Geometry: see drawing. Coordinates: mm, zero at the bounding-box minimum. A direction names the side the tool comes from. Coordinates: 2 decimals unless noted, no trailing zeros. Loops run counter-clockwise (first coordinate to the right, second up) from the corner with the lowest first, then second, coordinate; pieces in that order, holes last. Notation, with made-up numbers: (56.5, 32) -> (67.5, 32) arc R33 ccw to (67.5, 65) -> close; hole circle Ø10 at (-29, -24). An arc over 180 degrees is marked (long way). Put each result on its own line as item: value. Start each with the question number.
1) Contact query for flat-ended pins moving along their axis: P1, Ø1, axis at x = 2.5, z = 4, coming from the +Y side; P2, Ø1, axis at y = 3.5, z = 27, coming from the +X side; P3, Ø2, axis at x = 1, z = 13.5, coming from the -Y side; P4, Ø1, axis at y = 3, z = 24.5, coming from the -X side. Output: stop coordinate, or through.
2) Cut plane B-B (z = 9). Return the cut outline in (x, y).
3) Cut plane C-C (y = 3.85). Return the cut outline in (x, z).
4) Set-up query: the marked faces 1, 2 and 3. Return all of +Z, -Z, +X, -X, +Y, -Y with unobstructed straight access to the full face (end or side cutting, diameter ignored); none if empty.
5) Cut plane A-A (x = 2.65). Return the cut outline in (y, z).
6) Material intervals for L1, parallel to Z at x = 2.7, y = 5.1; L2, parallel to X at y = 4.5, z = 30, sorted ascending.
7) Cut plane D-D (x = 4.05). Return the cut outline in (y, z), plus the area to 3 significant figures.
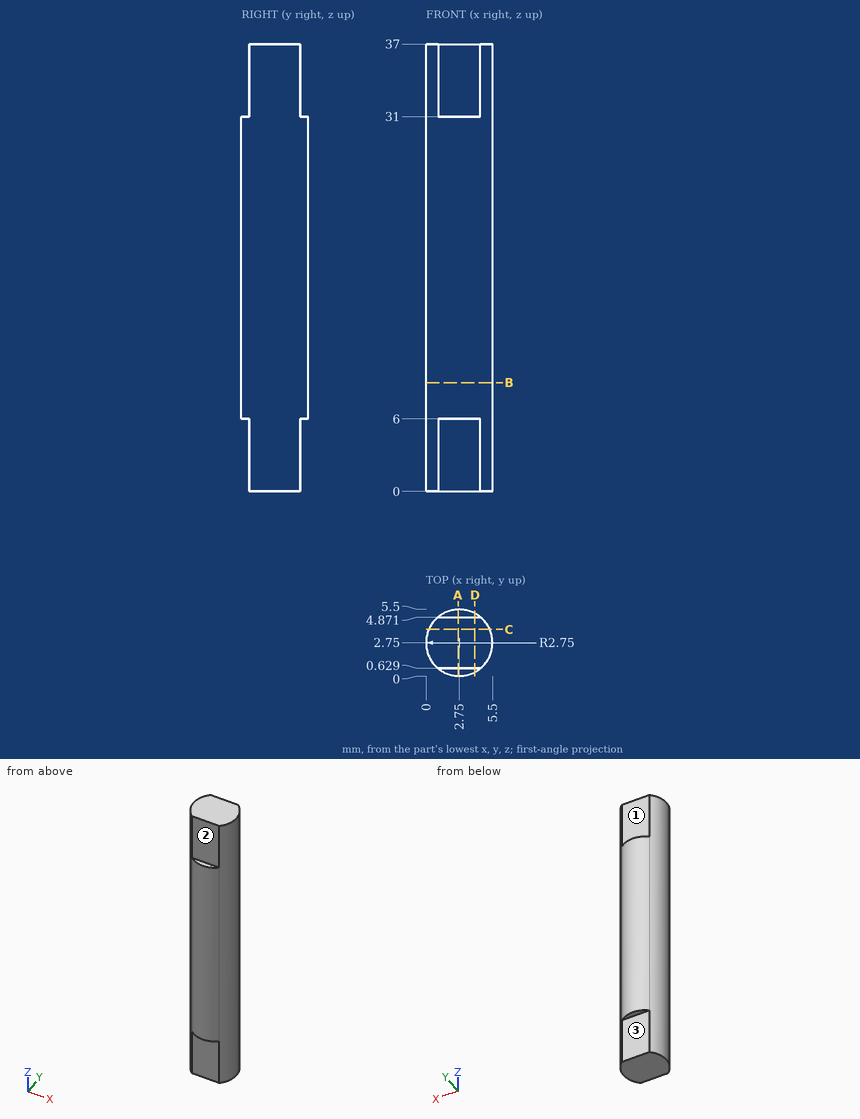
Results found:
1. P1: stops at y = 4.87
1. P2: stops at x = 5.49
1. P3: stops at y = 0.1
1. P4: stops at x = 0
2. outline: circle Ø5.5 at (2.75, 2.75)
3. outline: (0.23, 0) -> (5.27, 0) -> (5.27, 37) -> (0.23, 37) -> close
4. face 1: +Z, +X, -X, +Y
4. face 2: +Z, +X, -X, -Y
4. face 3: -Z, +X, -X, +Y
5. outline: (0, 6) -> (0.63, 6) -> (0.63, 0) -> (4.87, 0) -> (4.87, 6) -> (5.5, 6) -> (5.5, 31) -> (4.87, 31) -> (4.87, 37) -> (0.63, 37) -> (0.63, 31) -> (0, 31) -> close
6. L1: z = 6 to 31
6. L2: x = 0.63 to 4.87
7. outline: (0.33, 6) -> (0.63, 6) -> (0.63, 0) -> (4.87, 0) -> (4.87, 6) -> (5.17, 6) -> (5.17, 31) -> (4.87, 31) -> (4.87, 37) -> (0.63, 37) -> (0.63, 31) -> (0.33, 31) -> close
7. area: 172 mm2
